Job drawing, mm, ordinate dimensions from the low corner. One solid piece. Give positions to 0.01 mm unless a question says otherwise; leave off trailing zeros. Write each loop counter-clockwise with the first axis right and the second up, starting at its lowest first coordinate (ties: lowest second). Pieces come first, ordered by that corner, then holes. Notation, with made-up numbers: M 44,-19 L 89,-19 A13 cw 89,-11 Z; hole C -9,12 d8. An arc over 180 degrees is marked long. Answer as CSV lines item,"result". Start each with the question number.
1) Pin check, flat tips, straight feed: pin 1 Ø1.8 at (y, z) = (5, 115) entering from -X; pin 2 Ø5 at (x, z) = (8, 78) entering from -Y; pin 3 Ø5 at (x, z) = (5.5, 58.5) entering from -Y; pin 4 Ø6 at (y, z) = (1, 107) entering from -X. Stop position of each tip, or through.
2) Slice it at B-B, the plane x = 4. Give the cut face in (y, z).
3) Mould opens along Y. For the marked faces 1 and 2 say: pulls with the +Y half, pulls with the -Y half, needs draft (parallel to the pull), parting line crosses it, or undercut.
4) Wall check: line 1 along Y through (x, z) = (5.25, 5); line 2 along Z through (x, y) = (7, 7.75); line 3 along Y through (x, z) = (2.75, 5). Give the ranges that are in metal, low to high. Write a range as from..to.
5) Slice it at A-A, the plane x = 8.75. Give the cut face in (y, z), plus the area to 3 significant figures.
6) Slice it at D-D, the plane z = 56.5. Give the cut face in (x, y).
7) Slice it at C-C, the plane z = 115. Give the cut face in (x, y).
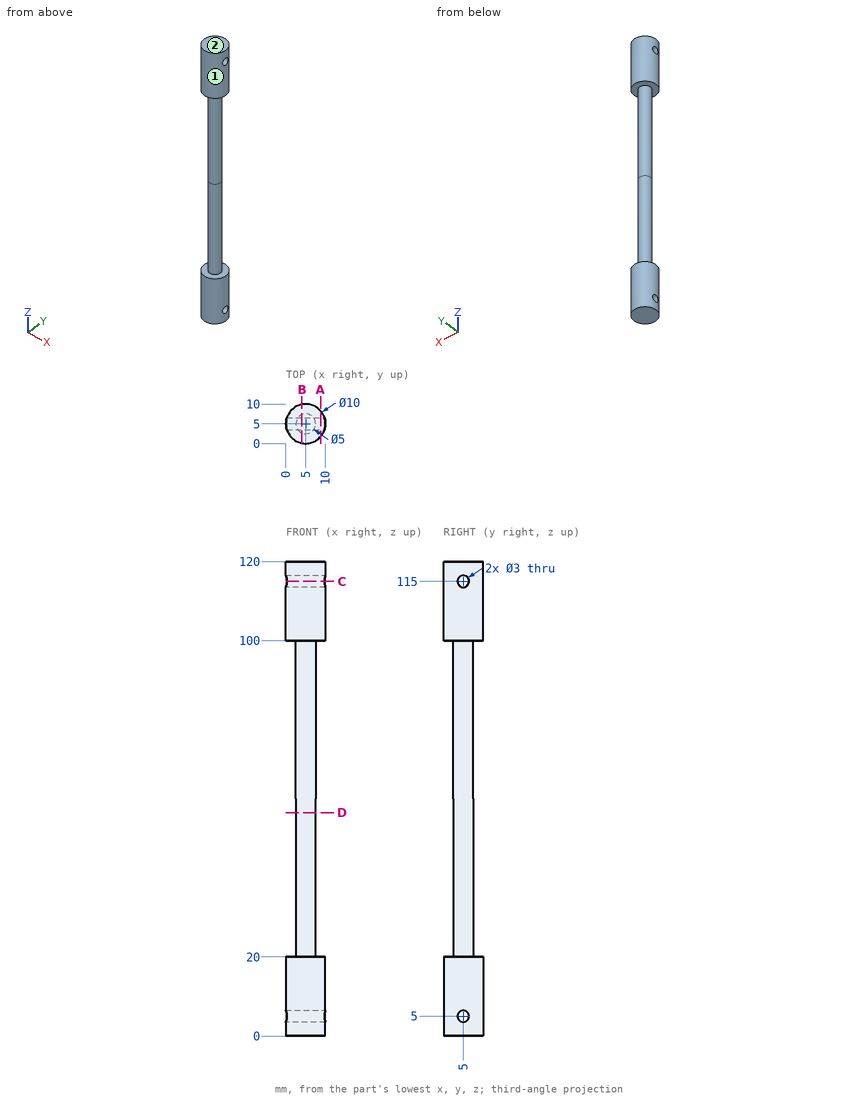
Found:
1,pin 1,"through"
1,pin 2,"y = 2.55"
1,pin 3,"y = 2.5"
1,pin 4,"x = 0.1"
2,outline,"M 0.1,0 L 9.9,0 L 9.9,20 L 7.29,20 L 7.29,100 L 9.9,100 L 9.9,120 L 0.1,120 L 0.1,100 L 2.71,100 L 2.71,20 L 0.1,20 Z; hole C 5,5 d3; hole C 5,115 d3"
3,face 1,"parting line crosses it"
3,face 2,"needs draft"
4,line 1,"0.01..3.5, 6.5..9.99"
4,line 2,"0..20, 100..120"
4,line 3,"0.53..3.5, 6.5..9.47"
5,outline,"M 1.69,0 L 8.31,0 L 8.31,20 L 1.69,20 Z; M 1.69,100 L 8.31,100 L 8.31,120 L 1.69,120 Z; hole C 5,5 d3; hole C 5,115 d3"
5,area,"250 mm²"
6,outline,"C 5,5 d5"
7,outline,"M 0.23,3.5 A5 ccw 9.77,3.5 Z; M 0.23,6.5 L 9.77,6.5 A5 ccw Z"
